Part model, mm, in its own coordinate system. Give positions to 0.01 mm unless a question says otherwise; leave off trailing zeros. Order: outer loops, then holes, each group sorted by start corner. A loop starts at its lowest first (then second) coordinate and runs counter-clockwise, first axis right, second up.
1. Slice it at A-A on y = 519. List the corners of the cut face in (x, z).
2. Slice it at B-B on z = 2.2. List the corners of the cut face in (x, y), and give its area (3 significant figures).
3. Drop flat-ended pins along their axis: pin 1 Ø2.5 at (x, y) = (1164.04, 548.89) entering from +Z; pin 2 Ø1 at (x, z) = (1183, 2.5) entering from +Y. Give the stop position or say it passes through.
4. Probe line 1 (X direction, y = 559.5, z = 0.2); line 2 (X direction, y = 534, z = 1.55); line 3 (X direction, y = 563, z = 1.85). List the from-to ranges inside material, lowest first.
5. Slice it at D-D on x = 1183.5. List the corners of the cut face in (y, z).
6. Mould opens along X. For faces 1 (the cylindrical face through (1146.59, 567.11, 1.48)), 2 (the cylindrical face through (1466.229, 578.276, 1.479)), 3 (the flat face through (1310, 498, 3)) say: +X half, -X half, draft (parallel to the pull), parting line (faces both ways), or undercut.
7. Slice it at C-C on x = 1395. List the corners of the cut face in (y, z), and give its area (3 significant figures).
from build123d import *

# Parameters (mm, degrees)
PAD014_DEPTH                        = 3
SKETCH055_R                         = 1.65
POCKET019_DEPTH                     = 364.282338
POCKET019_DEPTH_BACK                = 367.282338
BODY001003005003003_PLACEMENT_ANGLE = 60
CLONE003_PLACEMENT_ANGLE            = 122


with BuildPart() as part:
    # Sketch052 → Pad014 (new body)
    with BuildSketch(Plane.XY):
        with BuildLine():
            ThreePointArc((152.959511, 127.101705), (84.480895, 180.040089), (0, 198.875477))
            Line((0, 198.875477), (0, 208.875477))
            ThreePointArc((160.650731, 133.492724), (88.728824, 189.092995), (0, 208.875477))
            ThreePointArc((152.959511, 127.101705), (160.000631, 126.451604), (160.650731, 133.492724))
        make_face()
    pad014 = extrude(amount=PAD014_DEPTH)

    # Sketch055 → Pocket019 (cut, two sides)
    with BuildSketch(Plane.XY) as pocket019_sk:
        with Locations((143.11, 145.205847)):
            Circle(SKETCH055_R)
        with BuildLine():
            Line((0, 202.225477), (0, 205.525477))
            ThreePointArc((0, 202.225477), (1.65, 203.875477), (0, 205.525477))
        make_face()
    pocket019 = extrude(amount=-POCKET019_DEPTH, mode=Mode.SUBTRACT) + extrude(pocket019_sk.sketch, amount=POCKET019_DEPTH_BACK, mode=Mode.SUBTRACT)

    # Mirrored019: Pad014, Pocket019 across Sketch052 V_Axis
    add(pad014.mirror(Plane(origin=(0, 0, 0), x_dir=(0, 0, 1), z_dir=(1, 0, 0))))
    add(pocket019.mirror(Plane(origin=(0, 0, 0), x_dir=(0, 0, 1), z_dir=(1, 0, 0))), mode=Mode.SUBTRACT)


with BuildPart() as part_1:
    # Body001003005003003 placement: moved
    add(part.part.rotate(Axis((0, 0, 0), (0, 0, 1)), BODY001003005003003_PLACEMENT_ANGLE))


with BuildPart() as part_2:
    # Clone003 placement: moved
    add(part_1.part.moved(Location((1302, 699, 0))).rotate(Axis((1302, 699, 0), (0, 0, 1)), CLONE003_PLACEMENT_ANGLE))


solid = part_2.part
Data:
1. outline: (1196.03, 0) - (1217.43, 0) - (1217.43, 3) - (1196.03, 3) - close; (1386.57, 0) - (1407.97, 0) - (1407.97, 3) - (1386.57, 3) - close
2. outline: (1146.11, 559.98) arc R208.88 ccw to (1309.29, 490.25) arc R208.88 ccw to (1467.21, 571.2) arc R5 ccw to (1459.3, 577.31) arc R198.88 cw to (1308.94, 500.25) arc R198.88 cw to (1153.57, 566.64) arc R5 ccw to start; hole circle Ø3.3 at (1164.04, 548.89); hole circle Ø3.3 at (1309.12, 495.25); hole circle Ø3.3 at (1450.09, 558.88)
2. area: 3,630 mm2
3. pin 1: passes through
3. pin 2: stops at y = 540.03
4. line 1: x = 1146.54 to 1160.26, 1443.74 to 1448.56, 1451.62 to 1457.46
4. line 2: x = 1173.92 to 1190.98, 1413.02 to 1430.08
4. line 3: x = 1144.85 to 1156.9, 1447.1 to 1460.53
5. outline: (526.99, 0) - (539.28, 0) - (539.28, 3) - (526.99, 3) - close
6. face 1: undercut
6. face 2: parting line
6. face 3: draft
7. outline: (511.97, 0) - (523.21, 0) - (523.21, 3) - (511.97, 3) - close
7. area: 33.7 mm2
